```python
from build123d import *

# Parameters (mm, degrees)
PAD_DEPTH       = 4
SKETCH001_R     = 1.5
SKETCH001_R_2   = 2
SKETCH001_R_3   = 6
SKETCH001_W     = 5
SKETCH001_H     = 5
SKETCH001_W_2   = 10
SKETCH001_W_3   = 20
POCKET_DEPTH    = 5
SKETCH002_W     = 20
SKETCH002_H     = 4
POCKET001_DEPTH = 5
SKETCH003_W     = 4
SKETCH003_H     = 20
POCKET002_DEPTH = 5


with BuildPart() as part:
    # Sketch → Pad (new body)
    with BuildSketch(Plane.XZ):
        Polygon((0, 0), (240, 0), (240, 30), (220, 50), (0, 50), align=None)
    extrude(amount=PAD_DEPTH)

    # Sketch001 (on Face7 of Pad) → Pocket (cut)
    with BuildSketch(Plane.XZ.offset(4)):
        with Locations((16.976847, 24.364438)):
            Circle(SKETCH001_R)
        with Locations((24.976847, 15.364438)):
            Circle(SKETCH001_R_2)
        with Locations((35.976847, 15.364438)):
            Circle(SKETCH001_R_3)
        with Locations((16.976847, 6.364438)):
            Circle(SKETCH001_R)
        with Locations((5.976847, 15.364438)):
            Rectangle(SKETCH001_W, SKETCH001_H)
        with Locations((105, 47.5)):
            Rectangle(SKETCH001_W_2, SKETCH001_H)
        with Locations((140, 47.5)):
            Rectangle(SKETCH001_W_3, SKETCH001_H)
    extrude(amount=-POCKET_DEPTH, mode=Mode.SUBTRACT)

    # Sketch002 (on Face5 of Pocket) → Pocket001 (cut)
    with BuildSketch(Plane.XZ.offset(4)):
        with Locations((30, 2)):
            Rectangle(SKETCH002_W, SKETCH002_H)
        with Locations((70, 2)):
            Rectangle(SKETCH002_W, SKETCH002_H)
        with Locations((110, 2)):
            Rectangle(SKETCH002_W, SKETCH002_H)
        with Locations((150, 2)):
            Rectangle(SKETCH002_W, SKETCH002_H)
        with Locations((190, 2)):
            Rectangle(SKETCH002_W, SKETCH002_H)
        with Locations((230, 2)):
            Rectangle(SKETCH002_W, SKETCH002_H)
    extrude(amount=-POCKET001_DEPTH, mode=Mode.SUBTRACT)

    # Sketch003 (on Face4 of Pocket001) → Pocket002 (cut)
    with BuildSketch(Plane.XZ.offset(4)):
        with Locations((62, 40)):
            Rectangle(SKETCH003_W, SKETCH003_H)
    extrude(amount=-POCKET002_DEPTH, mode=Mode.SUBTRACT)


solid = part.part
```
Check sheet for the modelled part. Datum: model origin and axes. Units: mm. A direction names the side the tool comes from. Give positions to 0.01 mm unless a question says otherwise; leave off trailing zeros. Write each loop counter-clockwise with the first axis right and the second up, starting at its lowest first coordinate (ties: lowest second). Pieces come first, ordered by that corner, then holes. Notation, with made-up numbers: (15, 2) -> (59, 2) arc R10 cw to (59, 20) -> close; hole circle Ø6 at (44.25, 36.5). An arc over 180 degrees is marked (long way). Use CSV: the item, a comma, the result in double quotes. Start each with the question number.
Q1. Scan lines: line 1 along X through (y, z) = (-1.95, 17); line 2 along X through (y, z) = (-2.9, 6); line 3 along X through (y, z) = (-1.95, 45.5). Record each from-to range of solid material in increasing order.
Q2. Cross-section at B-B on z = 47. Enter the section's corners in (x, y), and give its area (3 significant figures).
Q3. Cross-section at A-A on z = 32. Enter the section's corners in (x, y).
Q4. Cross-section at D-D on y = -3.3. Count the separate pieces of the cut face and the enclosed holes in it, and give its area (3 significant figures).
Q5. Release check for a two-part mould opening along X. For faces 4 (the flat face through (0, -2, 25)), 5 (the flat face through (80, -2, 2)), 6 (the flat face through (82, -2, 50)) record: +X half, -X half, draft (parallel to the pull), parting line (faces both ways), or undercut.
Q6. Depth check by flat-ended pin: P1, Ø1.2, axis at x = 192, y = -1.5, coming from the -Z side; P2, Ø2, axis at x = 105.5, y = -1.5, coming from the +Z side; P3, Ø1.2, axis at y = -1.5, z = 2, coming from the +X side; P4, Ø3, axis at x = 24.98, z = 15.36, coming from the +Y side. Enter the tip coordinate at first touch or a pass-through.
Q7. Tool access check on faces 1 (the flat face through (60, -2, 40)), 2 (the flat face through (20, -2, 2)), 3 (the flat face through (185, -2, 50)). Record the directions out of +Z, -Z, +X, -X, +Y, -Y that give a thin tool (end or side, any length) a straight path to the whole face; none if there is none.
Q8. Cross-section at C-C on x = 187. Enter the section's corners in (y, z), and give its area (3 significant figures).
Working result:
1,line 1,"x = 0 to 3.48, 8.48 to 23.83, 26.13 to 30.2, 41.75 to 240"
1,line 2,"x = 0 to 15.52, 18.43 to 240"
1,line 3,"x = 0 to 60, 64 to 100, 110 to 130, 150 to 224.5"
2,outline,"(0, -4) -> (60, -4) -> (60, 0) -> (0, 0) -> close; (64, -4) -> (100, -4) -> (100, 0) -> (64, 0) -> close; (110, -4) -> (130, -4) -> (130, 0) -> (110, 0) -> close; (150, -4) -> (223, -4) -> (223, 0) -> (150, 0) -> close"
2,area,"756 mm^2"
3,outline,"(0, -4) -> (60, -4) -> (60, 0) -> (0, 0) -> close; (64, -4) -> (238, -4) -> (238, 0) -> (64, 0) -> close"
4,separate pieces,"1"
4,enclosed holes,"5"
4,area,"10,900 mm^2"
5,face 4,"-X half"
5,face 5,"undercut"
5,face 6,"draft"
6,P1,"stops at z = 4"
6,P2,"stops at z = 45"
6,P3,"stops at x = 220"
6,P4,"passes through"
7,face 1,"+Z, +Y, -Y"
7,face 2,"-Z, +Y, -Y"
7,face 3,"+Z, +X, -X, +Y, -Y"
8,outline,"(-4, 4) -> (0, 4) -> (0, 50) -> (-4, 50) -> close"
8,area,"184 mm^2"
